Read the model definition and answer for the solid it produces. Units are mm, in the model's axes. Face numbers are marked on the shaded views. Coordinates: 2 decimals unless noted, no trailing zeros. Loops run counter-clockwise (first coordinate to the right, second up) from the corner with the lowest first, then second, coordinate; pieces in that order, holes last. Notation, with made-up numbers: (-21.5, 46) -> (37.5, 46) arc R28 cw to (37.5, 70) -> close; hole circle Ø7 at (76.25, 82). An arc over 180 degrees is marked (long way). Answer as a JSON object with one key per item and string values. Group by question number.
1) Determine the mould class of the marked faces 1, 2 and 3 for opening direction Y: released by +Y, released by -Y, zero draft, split by the parting line, or undercut.
2) Consider probe 1 along Y at (x, z) = (1, 3.5); probe 2 along Z at (x, y) = (5, -9.25); probe 3 along Z at (x, y) = (4.5, -6.5). Determine where each line is inside the solid, lowest interval first. Write a range as [from, to].
3) Section A-A, the plane x = -8.5 is taken. Give the vertices of the cut face in (y, z), plus the area to 3 significant figures.
4) Flat-ended cylindrical pins translate along their axes: P1, Ø6, axis at x = -12, y = -8.5, coming from the +Z side; P2, Ø12, axis at y = -7.5, z = 25.5, coming from the -X side; P3, Ø12, axis at x = -20, y = 1.5, coming from the -Z side. Find the tip coordinate at first contact, or state that the pin passes through.
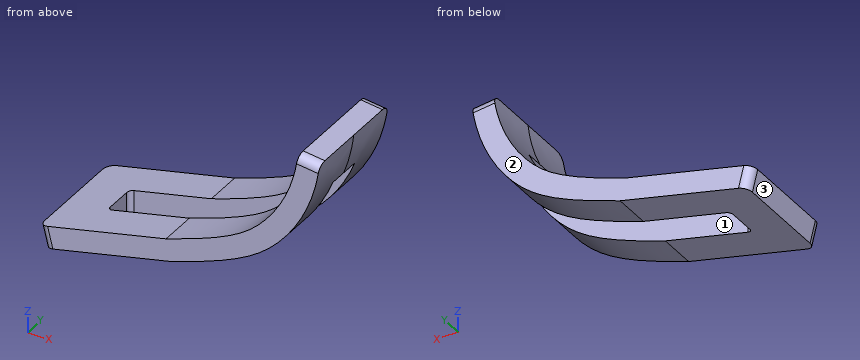
from build123d import *

# Parameters (mm, degrees)
F1_DEPTH      = 12.5
F1_DEPTH_BACK = 12.5
F2_R          = 2
F4_DEPTH      = 25
F4_DEPTH_BACK = 25


# Not quite as in the source:
# - ends of sketch curves that miss each other by under 0.0002 mm in the source are joined
# - the dataset's text gives a spline's control points without its knots; the knots are read off the source's solid


with BuildPart() as f1:
    # F0 (on Front) → F1 (new body, two sides)
    with BuildSketch(Plane.XZ) as f1_sk:
        with BuildLine():
            Line((-1.2184032821, 4.8688166534), (0, 0))
            add(Edge.make_bspline(
                [(0, 0), (13.9942302595, 4.8154504329), (25.3093838267, 10.870907846), (33.031907279, 25.9106602745), (33.9476719961, 34.5905660178)],
                knots=[0, 0, 0, 0, 0.5280763551, 1, 1, 1, 1], degree=3))
            Line((33.9476719961, 34.5905660178), (28.975269547, 35.1151743323))
            add(Edge.make_bspline(
                [(-1.2184032821, 4.8688166534), (1.8648217541, 5.9349029149), (7.287113618, 7.9315285829), (12.1983004489, 10.1724794599), (15.2865186932, 11.9439955294), (17.2413608312, 13.281183998), (18.9416466936, 14.6787902185), (20.2373870468, 15.9523435041), (21.2534611324, 17.0823993837), (22.2542990458, 18.283251609), (23.9332185037, 20.5443961427), (26.0676758341, 24.2225990158), (28.0070847052, 29.2983814533), (28.7632711893, 33.1057872835), (28.975269547, 35.1151743323)],
                knots=[0.0052558834, 0.0052558834, 0.0052558834, 0.0052558834, 0.125, 0.25, 0.3125, 0.375, 0.4375, 0.5, 0.53125, 0.5625, 0.625, 0.75, 0.875, 1, 1, 1, 1], degree=3))
        make_face()
        Polygon((-29.1025877416, -7.2828144797), (0, 0), (-1.2184032821, 4.8688166534), (-30.3209910237, -2.4139978263), align=None)
    extrude(amount=F1_DEPTH)
    extrude(f1_sk.sketch, amount=-F1_DEPTH_BACK)

    # F2
    f2_edges = [f1.edges().sort_by_distance(p)[0] for p in [
        (31.461471, -12.5, 34.85287),
        (31.461471, 12.5, 34.85287),
        (-29.711789, -12.5, -4.848406),
        (-29.711789, 12.5, -4.848406),
    ]]
    fillet(f2_edges, radius=F2_R)

    # F3 (on Top) → F4 (cut, two sides)
    with BuildSketch(Plane.XY) as f4_sk:
        with BuildLine():
            Line((-19, -4), (50, -4))
            Line((50, -4), (50, 4))
            Line((50, 4), (-19, 4))
            ThreePointArc((-19, 4), (-19.7071067812, 3.7071067812), (-20, 3))
            Line((-20, 3), (-20, -3))
            ThreePointArc((-20, -3), (-19.7071067812, -3.7071067812), (-19, -4))
        make_face()
    extrude(amount=F4_DEPTH, mode=Mode.SUBTRACT)
    extrude(f4_sk.sketch, amount=-F4_DEPTH_BACK, mode=Mode.SUBTRACT)


solid = f1.part
Determined:
{
 "1": {"face 1": "undercut", "face 2": "released by +Y", "face 3": "zero draft"},
 "2": {"probe 1": "[-12.5, -4], [4, 12.5]", "probe 2": "[1.78, 7.12]", "probe 3": "[1.6, 6.93]"},
 "3": {"outline": "(-12.5, -2.13) -> (-4, -2.13) -> (-4, 3.05) -> (-12.5, 3.05) -> close; (4, -2.13) -> (12.5, -2.13) -> (12.5, 3.05) -> (4, 3.05) -> close", "area": "88.0 mm²"},
 "4": {"P1": "z = 2.92", "P2": "x = 23.14", "P3": "z = -6.51"}
}
